```python
from build123d import *

# Parameters (mm, degrees)
SKETCH_1_R      = 1.7
SKETCH_1_R_2    = 3.25
EXTRUDE_1_DEPTH = 3


with BuildPart() as part:
    # 草图1 → 凸台-拉伸1 (new body)
    with BuildSketch(Plane.XY):
        with BuildLine():
            Line((-13.46, 3.883091552), (-1.68, 6.795410216))
            ThreePointArc((-1.68, 6.795410216), (0, 7), (1.68, 6.795410216))
            Line((1.68, 6.795410216), (13.46, 3.883091552))
            ThreePointArc((13.46, 3.883091552), (16.5, 0), (13.46, -3.883091552))
            Line((13.46, -3.883091552), (1.68, -6.795410216))
            ThreePointArc((1.68, -6.795410216), (0, -7), (-1.68, -6.795410216))
            Line((-1.68, -6.795410216), (-13.46, -3.883091552))
            ThreePointArc((-13.46, -3.883091552), (-16.5, 0), (-13.46, 3.883091552))
        make_face()
        with Locations((-12.5, 0)):
            Circle(SKETCH_1_R, mode=Mode.SUBTRACT)
        Circle(SKETCH_1_R_2, mode=Mode.SUBTRACT)
        with Locations(Location((12.5, 0, 0), (0, 0, 180))):
            Circle(SKETCH_1_R, mode=Mode.SUBTRACT)
    extrude(amount=EXTRUDE_1_DEPTH)


solid = part.part
```
Work out the finished part from the listing and answer in its coordinate system (mm). Round coordinates to 2 decimals unless told otherwise and drop trailing zeros. Loops run counter-clockwise (first coordinate to the right, second up) from the corner with the lowest first, then second, coordinate; pieces in that order, holes last.
(1) The mould has two halves that part along X. Classify faces 1 (the flat face through (-7.49, -5.36, 1.48)), 2 (the cylindrical face through (10.93, 0.65, 1.48)), 3 (the cylindrical face through (-10.93, -0.65, 1.48)), 4 (the cylindrical face through (0, 7, 1)): pulls with the +X half, pulls with the -X half, needs draft (parallel to the pull), parting line crosses it, or undercut.
Computed values:
face 1: pulls with the -X half
face 2: undercut
face 3: undercut
face 4: parting line crosses it
(2) The part is cut by section C-C, the plane z = 1.5. Give the vertices of the cut face in (x, y).
Computed values:
outline: (-13.46, -3.88) - (-1.68, -6.8) arc R7 ccw to (1.68, -6.8) - (13.46, -3.88) arc R4 ccw to (13.46, 3.88) - (1.68, 6.8) arc R7 ccw to (-1.68, 6.8) - (-13.46, 3.88) arc R4 ccw to start; hole circle Ø3.4 at (-12.5, 0); hole circle Ø6.5 at (0, 0); hole circle Ø3.4 at (12.5, 0)
(3) Each of these flat-tipped pins is pushed along its axis until it touches: P1, Ø2.5, axis at x = 12.5, y = 0, coming from the -Z side; P2, Ø4, axis at x = -2.5, y = 1, coming from the -Z side; P3, Ø1, axis at y = -1.5, z = 1.5, coming from the +X side. Where does it stop, or does it pass through?
Computed values:
P1: passes through
P2: stops at z = 0
P3: stops at x = 16.37
(4) The part is cut by section D-D, the plane y = 2.5. Give the vertices of the cut face in (x, z), and give its area (3 significant figures).
Computed values:
outline: (-15.62, 0) - (-2.08, 0) - (-2.08, 3) - (-15.62, 3) - close; (2.08, 0) - (15.62, 0) - (15.62, 3) - (2.08, 3) - close
area: 81.3 mm2
(5) The part is cut by section A-A, the plane x = 0. Give the vertices of the cut face in (y, z), and give its area (3 significant figures).
Computed values:
outline: (-7, 0) - (-3.25, 0) - (-3.25, 3) - (-7, 3) - close; (3.25, 0) - (7, 0) - (7, 3) - (3.25, 3) - close
area: 22.5 mm2
(6) The part is cut by section B-B, the plane y = 0. Give the vertices of the cut face in (x, z), and give its area (3 significant figures).
Computed values:
outline: (-16.5, 0) - (-14.2, 0) - (-14.2, 3) - (-16.5, 3) - close; (-10.8, 0) - (-3.25, 0) - (-3.25, 3) - (-10.8, 3) - close; (3.25, 0) - (10.8, 0) - (10.8, 3) - (3.25, 3) - close; (14.2, 0) - (16.5, 0) - (16.5, 3) - (14.2, 3) - close
area: 59.1 mm2
(7) Find the intervals of material crossed by L1, parallel to Y at x = 0, z = 1.65; L2, parallel to X at y = -0.25, z = 2.3; L3, parallel to X at y = -2.5, z = 1.4, in increasing order.
Computed values:
L1: y = -7 to -3.25, 3.25 to 7
L2: x = -16.49 to -14.18, -10.82 to -3.24, 3.24 to 10.82, 14.18 to 16.49
L3: x = -15.62 to -2.08, 2.08 to 15.62
